```python
from build123d import *

# Parameters (mm, degrees)
CROQUIS1_R              = 1.5
CROQUIS1_R_2            = 15
SALIENTE_EXTRUIR1_DEPTH = 31.55


with BuildPart() as part:
    # Croquis1 → Saliente-Extruir1 (new body)
    with BuildSketch(Plane(origin=(0, 31.55, 0), x_dir=(1, 0, 0), z_dir=(0, 1, 0))):
        with BuildLine():
            Line((-12.857359313, -21), (12.857359313, -21))
            ThreePointArc((12.857359313, -21), (14.00540961, -20.771638598), (14.978679656, -20.121320344))
            Line((14.978679656, -20.121320344), (20.121320344, -14.978679656))
            ThreePointArc((20.121320344, -14.978679656), (20.771638598, -14.00540961), (21, -12.857359313))
            Line((21, -12.857359313), (21, 12.857359313))
            ThreePointArc((21, 12.857359313), (20.771638598, 14.00540961), (20.121320344, 14.978679656))
            Line((20.121320344, 14.978679656), (14.978679656, 20.121320344))
            ThreePointArc((14.978679656, 20.121320344), (14.00540961, 20.771638598), (12.857359313, 21))
            Line((12.857359313, 21), (-12.857359313, 21))
            ThreePointArc((-12.857359313, 21), (-14.00540961, 20.771638598), (-14.978679656, 20.121320344))
            Line((-14.978679656, 20.121320344), (-20.121320344, 14.978679656))
            ThreePointArc((-20.121320344, 14.978679656), (-20.771638598, 14.00540961), (-21, 12.857359313))
            Line((-21, 12.857359313), (-21, -12.857359313))
            ThreePointArc((-21, -12.857359313), (-20.771638598, -14.00540961), (-20.121320344, -14.978679656))
            Line((-20.121320344, -14.978679656), (-14.978679656, -20.121320344))
            ThreePointArc((-14.978679656, -20.121320344), (-14.00540961, -20.771638598), (-12.857359313, -21))
        make_face()
        with Locations(Location((15.5, -15.5, 0), (0, 0, 90))):
            Circle(CROQUIS1_R, mode=Mode.SUBTRACT)
        with Locations(Location((0, 0, 0), (0, 0, 90))):
            Circle(CROQUIS1_R_2, mode=Mode.SUBTRACT)
        with Locations(Location((15.5, 15.5, 0), (0, 0, 90))):
            Circle(CROQUIS1_R, mode=Mode.SUBTRACT)
        with Locations(Location((-15.5, -15.5, 0), (0, 0, 90))):
            Circle(CROQUIS1_R, mode=Mode.SUBTRACT)
        with Locations(Location((-15.5, 15.5, 0), (0, 0, 90))):
            Circle(CROQUIS1_R, mode=Mode.SUBTRACT)
    extrude(amount=-SALIENTE_EXTRUIR1_DEPTH)


solid = part.part
```
Read the model definition and answer for the solid it produces. Units are mm, in the model's axes. Round coordinates to 2 decimals unless told otherwise and drop trailing zeros. Write each loop counter-clockwise with the first axis right and the second up, starting at its lowest first coordinate (ties: lowest second). Pieces come first, ordered by that corner, then holes. Notation, with made-up numbers: M -2,63 L 47,63 A12 cw 47,71 Z; hole C 65.25,-19 d4. An arc over 180 degrees is marked long. One line per item, written item: value.
Q1. Find section A-A on x = 0. Write down the section's boundary in (y, z), plus the area to 3 significant figures.
Data:
outline: M 0,-21 L 31.55,-21 L 31.55,-15 L 0,-15 Z; M 0,15 L 31.55,15 L 31.55,21 L 0,21 Z
area: 379 mm2
Q2. Flat-ended cylindrical pins translate along their axes: pin 1 Ø4 at (x, y) = (-16, 6.5) entering from -Z; pin 2 Ø1 at (y, z) = (4, 16.5) entering from -X. Find the tip coordinate at first contact, or state that the pin passes through.
Data:
pin 1: z = -20.77
pin 2: x = -19.1
Q3. Find section B-B on y = 10.5. Write down the section's boundary in (x, z).
Data:
outline: M -21,-12.86 A3 ccw -20.12,-14.98 L -14.98,-20.12 A3 ccw -12.86,-21 L 12.86,-21 A3 ccw 14.98,-20.12 L 20.12,-14.98 A3 ccw 21,-12.86 L 21,12.86 A3 ccw 20.12,14.98 L 14.98,20.12 A3 ccw 12.86,21 L -12.86,21 A3 ccw -14.98,20.12 L -20.12,14.98 A3 ccw -21,12.86 Z; hole C -15.5,-15.5 d3; hole C -15.5,15.5 d3; hole C 0,0 d30; hole C 15.5,-15.5 d3; hole C 15.5,15.5 d3
Q4. Find section D-D on z = 16. Write down the section's boundary in (x, y), plus the area to 3 significant figures.
Data:
outline: M -19.1,0 L -16.91,0 L -16.91,31.55 L -19.1,31.55 Z; M -14.09,0 L 14.09,0 L 14.09,31.55 L -14.09,31.55 Z; M 16.91,0 L 19.1,0 L 19.1,31.55 L 16.91,31.55 Z
area: 1,030 mm2
Q5. Straight lines are drawn through the part: line 1 (X direction, y = 24, z = -0.5); line 2 (X direction, y = 8.5, z = -15.5); line 3 (X direction, y = 20.5, z = -4). For each, find the intervals that lie inside material, in ascending order. Write a range as [from, to].
Data:
line 1: [-21, -14.99], [14.99, 21]
line 2: [-19.6, -17], [-14, 14], [17, 19.6]
line 3: [-21, -14.46], [14.46, 21]
Q6. For a pull along Z with two mould halves and no side action, classify faces 1 (the cylindrical face through (-20.78, 16, 13.99)), 2 (the flat face through (-21, 16, 0)), 3 (the cylindrical face through (-15.57, 16, 17)) as +Z half, -Z half, draft (parallel to the pull), parting line (faces both ways), or undercut.
Data:
face 1: +Z half
face 2: draft
face 3: undercut
Q7. Find section C-C on z = 0. Write down the section's boundary in (x, y).
Data:
outline: M -21,0 L -15,0 L -15,31.55 L -21,31.55 Z; M 15,0 L 21,0 L 21,31.55 L 15,31.55 Z
